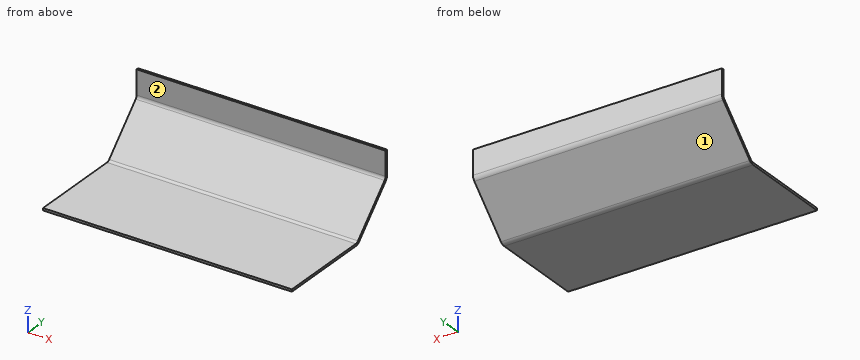
Autodesk Inventor part; units mm, degrees
ref_plane "YZ Plane" through (0, 0, 0) normal (1, 0, 0) x (0, 1, 0)
ref_plane "XZ Plane" through (0, 0, 0) normal (0, 1, 0) x (-1, 0, 0)
ref_plane "XY Plane" through (0, 0, 0) normal (0, 0, 1) x (1, 0, 0)
sketch "Sketch1" plane through (0, 0, 0) normal (0, 0, 1) x (1, 0, 0)
  line L0 (0, 0) -> (1100, 0)
  line L1 (1100, 0) -> (1100, 430)
  line L2 (1100, 430) -> (0, 430)
  line L3 (0, 430) -> (0, 0)
  dimension "d0" = 1100
  dimension "d1" = 430
extrude "Plate1" add sketch "Sketch1" along normal blind 10
sketch "Sketch2" plane through (0, 422.9289, 7.0711) normal (0, 0.7071068, -0.7071068) x (-1, 0, 0)
  line L0 (-1100, 0) -> (0, 0)
  line L1 (0, 0) -> (0, 270)
  line L2 (0, 270) -> (-1100, 270)
  line L3 (-1100, 270) -> (-1100, 0)
edge flange "Flange1" height 270 angle 45 thickness 10 bend radius 20 thickness toward (0, 0.7071068, -0.7071068) relief tear relief width 10 relief depth 5 edges at (550, 430, 10) wall of the first edge with corners at (1100, 422.9289, 7.0711) (0, 422.9289, 7.0711) (0, 613.8478, 197.9899) (1100, 613.8478, 197.9899)
bend "Bend1"
corner "Corner1"
sketch "Sketch3" plane through (0, 610.9188, 190.9188) normal (0, 1, 0) x (-1, 0, 0)
  line L0 (-1100, 0) -> (0, 0)
  line L1 (0, 0) -> (0, 120)
  line L2 (0, 120) -> (-1100, 120)
  line L3 (-1100, 120) -> (-1100, 0)
edge flange "Flange2" height 120 angle 45 thickness 10 bend radius 20 thickness toward (0, 1, 0) relief tear relief width 10 relief depth 5 edges at (550, 613.8478, 197.9899) wall of the first edge with corners at (1100, 610.9188, 190.9188) (0, 610.9188, 190.9188) (0, 610.9188, 310.9188) (1100, 610.9188, 310.9188)
bend "Bend2"
corner "Corner2"
equation "\"d2\" = Thickness"
equation "\"d3\" = BendReliefWidth"
equation "\"d4\" = BendReliefDepth"
equation "\"d5\" = MinimumRemnant"
equation "\"d6\" = TransitionRadius"
equation "\"d10\" = CornerReliefSize"
equation "\"d11\" = GapSize"
equation "\"d12\" = JacobiRadiusSize"
equation "\"d13\" = BendReliefWidth"
equation "\"d14\" = BendReliefDepth"
equation "\"d15\" = MinimumRemnant"
equation "\"d16\" = TransitionRadius"
equation "\"d20\" = CornerReliefSize"
equation "\"d21\" = GapSize"
equation "\"d22\" = JacobiRadiusSize"
equation "\"BendReliefDepth\" = 0.5 * Thickness"
properties part number "10mm Polycarb" material "Polycarbonate, Clear"
Source: CAD feature listing. Evaluate the final solid. Frame: model axes, mm. Face numbers are marked on the shaded views. A direction names the side the tool comes from. Give positions to 0.01 mm unless a question says otherwise; leave off trailing zeros. Write each loop counter-clockwise with the first axis right and the second up, starting at its lowest first coordinate (ties: lowest second). Pieces come first, ordered by that corner, then holes. Notation, with made-up numbers: (-3.5, 48) - (1.5, 48) arc R26 cw to (1.5, 82) - close; hole circle Ø1 at (5.25, 31.5). An arc over 180 degrees is marked (long way). One line per item, written item: value. Start each with the question number.
Q1. Section query C-C, the plane y = 124. Return the cut outline in (x, z).
Q2. Section query B-B, the plane z = 280.5. Return the cut outline in (x, y), then the cut area to 3 significant figures.
Q3. Set-up query: the marked faces 1 and 2. Return all of +Z, -Z, +X, -X, +Y, -Y with unobstructed straight access to the full face (end or side cutting, diameter ignored); none if empty.
Q4. First-contact query: pin 1 Ø10 at (x, y) = (802.5, 318.5) entering from +Z; pin 2 Ø12 at (x, z) = (445.5, 233.5) entering from -Y; pin 3 Ø5 at (x, z) = (523.5, 124.5) entering from +Y. Flat tips, straight axial feed; report the tip coordinate or a pass-through.
Q5. Material intervals for probe 1 along Y at (x, z) = (60.5, 205); probe 2 along Z at (x, y) = (602.5, 398); probe 3 along Y at (x, z) = (473, 175), sorted ascending. Write a range as from..to.
Q6. Section query A-A, the plane x = 103.5. Return the cut outline in (y, z).
Answer:
1. outline: (0, 0) - (1100, 0) - (1100, 10) - (0, 10) - close
2. outline: (0, 610.92) - (1100, 610.92) - (1100, 620.92) - (0, 620.92) - close
2. area: 11,000 mm2
3. face 1: -Z, +X, -X, +Y
3. face 2: +Z, +X, -X, -Y
4. pin 1: stops at z = 10
4. pin 2: stops at y = 610.92
4. pin 3: stops at y = 557
5. probe 1: y = 610.92..620.92
5. probe 2: z = 0..10
5. probe 3: y = 590.86..605
6. outline: (0, 0) - (417.57, 0) arc R30 ccw to (438.79, 8.79) - (612.13, 182.13) arc R30 ccw to (620.92, 203.35) - (620.92, 310.92) - (610.92, 310.92) - (610.92, 203.35) arc R20 cw to (605.06, 189.2) - (431.72, 15.86) arc R20 cw to (417.57, 10) - (0, 10) - close
